The listing builds one solid part. Answer for the finished solid, in the listing's coordinates (mm). A direction names the side the tool comes from. Round coordinates to 2 decimals unless told otherwise and drop trailing zeros. Order: outer loops, then holes, each group sorted by start corner. A loop starts at its lowest first (then second) coordinate and runs counter-clockwise, first axis right, second up. Notation, with made-up numbers: (44.5, 39.5) -> (59.5, 39.5) arc R13 cw to (59.5, 62.5) -> close; hole circle Ø4 at (48.5, -6.5). An arc over 180 degrees is marked (long way). Return JSON: item names as keys, results as strings. Group by question number.
(1) Each of these flat-tipped pins is pushed along its axis until it touches: pin 1 (1.5 mm diameter, centred on x = 53.5, y = 36, fed in from +Z); pin 2 (24.5 mm diameter, centred on x = 17.5, y = 17.5, fed in from +Z); pin 3 (5 mm diameter, centred on x = 8, y = 30.5, fed in from -Z). Where does it stop, or does it pass through?
(2) Consider line 1 (X direction, y = 4, z = 15.75); line 2 (Y direction, x = 26, z = 19); line 3 (Y direction, x = 21, z = 12.25). Determine where each line is inside the solid, lowest interval first. Write a range as [from, to].
(3) Determine the mould class of faces 1 (the face through (58.55, 15, 1)), 2 (the face through (57.05, 7, 11)), 3 (the face through (-2, 30, 16)) for opening direction X: +X half, -X half, draft (parallel to the pull), parting line (faces both ways), or undercut.
(4) The part is cut by section B-B (y = 9). Determine the outline of the cut face in (x, z), plus the area to 3 significant figures.
(5) The part is cut by section D-D (y = 19.5). Determine the outline of the cut face in (x, z).
(6) The part is cut by section A-A (x = 42.5). Determine the outline of the cut face in (y, z), plus the area to 3 significant figures.
(7) Which of the six approach directions +Z, -Z, +X, -X, +Y, -Y give full straight-line access (tool end or side, diameter ignored) to faces 4 (the face through (41, 49, 16)), 5 (the face through (29, 13.5, 10)), 6 (the face through (61, 45, 16))?
(8) The part is cut by section C-C (z = 8). Count the separate pieces of the cut face and the enclosed holes in it, plus the area to 3 significant figures.
from build123d import *

# Parameters (mm, degrees)
SKETCH1_W            = 64.05
SKETCH1_H            = 52.6
BOSS_EXTRUDE1_DEPTH  = 2
SKETCH2_W            = 64.05
SKETCH2_H            = 52.6
SKETCH2_W_2          = 60.05
SKETCH2_H_2          = 48.6
BOSS_EXTRUDE2_DEPTH  = 18
SKETCH3_W            = 64.05
SKETCH3_H            = 52.6
SKETCH3_W_2          = 62.45
SKETCH3_H_2          = 51
BOSS_EXTRUDE3_DEPTH  = 2.2
SKETCH6_W            = 52.55
SKETCH6_H            = 16
CUT_EXTRUDE2_DEPTH   = 15
BOSS_EXTRUDE4_DEPTH  = 18
CUT_EXTRUDE3_DEPTH   = 3
LPATTERN1_COUNT      = 8
LPATTERN1_PITCH      = 7.6
CUT_EXTRUDE4_DEPTH   = 3
LPATTERN2_COUNT      = 5
LPATTERN2_PITCH      = 7.6
MIRROR1_COPY_1_DEPTH = 3
MIRROR1_COPY_2_DEPTH = 3
MIRROR1_COPY_3_DEPTH = 3
MIRROR1_COPY_4_DEPTH = 3
FILLET1_R            = 1
SKETCH10_W           = 52.55
SKETCH10_H           = 30
CUT_EXTRUDE5_DEPTH   = 0.2
FILLET2_R            = 2


with BuildPart() as part:
    # Sketch1 → Boss-Extrude1 (new body)
    with BuildSketch(Plane.XY):
        with Locations((29.525, 23.8)):
            Rectangle(SKETCH1_W, SKETCH1_H)
    extrude(amount=BOSS_EXTRUDE1_DEPTH)

    # Sketch2 → Boss-Extrude2 (add)
    with BuildSketch(Plane.XY.offset(2)):
        with Locations((29.525, 23.8)):
            Rectangle(SKETCH2_W, SKETCH2_H)
        with Locations((29.525, 23.8)):
            Rectangle(SKETCH2_W_2, SKETCH2_H_2, mode=Mode.SUBTRACT)
    extrude(amount=BOSS_EXTRUDE2_DEPTH)

    # Sketch3 → Boss-Extrude3 (add)
    with BuildSketch(Plane.XY.offset(20)):
        with Locations((29.525, 23.8)):
            Rectangle(SKETCH3_W, SKETCH3_H)
        with Locations((29.525, 23.8)):
            Rectangle(SKETCH3_W_2, SKETCH3_H_2, mode=Mode.SUBTRACT)
    extrude(amount=BOSS_EXTRUDE3_DEPTH)

    # Sketch6 → Cut-Extrude2 (cut)
    with BuildSketch(Plane(origin=(0, 0, 0), x_dir=(-1, 0, 0), z_dir=(0, 0, -1))):
        with Locations((-29.775, 5.5)):
            Rectangle(SKETCH6_W, SKETCH6_H)
    extrude(amount=-CUT_EXTRUDE2_DEPTH, mode=Mode.SUBTRACT)

    # Sketch7 → Boss-Extrude4 (add)
    with BuildSketch(Plane.XY.offset(2)):
        Polygon((56.05, 13.5), (56.05, -0.5), (57.05, -0.5), (57.05, 14.5), (2.5, 14.5), (2.5, -0.5), (3.5, -0.5), (3.5, 13.5), align=None)
    extrude(amount=BOSS_EXTRUDE4_DEPTH)

    # Sketch8 → Cut-Extrude3 (cut)
    with BuildSketch(Plane(origin=(0, 50.1, 0), x_dir=(1, 0, 0), z_dir=(0, 1, 0))):
        Polygon((1.5, 0), (3.5, 0), (3.3, -16), (1.7, -16), align=None)
    cut_extrude3 = extrude(amount=-CUT_EXTRUDE3_DEPTH, mode=Mode.SUBTRACT)

    # LPattern1: Cut-Extrude3 ×8
    with Locations(*[(i * LPATTERN1_PITCH, 0, 0) for i in range(1, LPATTERN1_COUNT)]):
        add(cut_extrude3, mode=Mode.SUBTRACT)

    # Sketch9 → Cut-Extrude4 (cut)
    with BuildSketch(Plane(origin=(61.55, 0, 0), x_dir=(0, 0, -1), z_dir=(1, 0, 0))):
        Polygon((0, 46.1), (0, 44.1), (-16, 44.3), (-16, 45.9), align=None)
    cut_extrude4 = extrude(amount=-CUT_EXTRUDE4_DEPTH, mode=Mode.SUBTRACT)

    # LPattern2: Cut-Extrude4 ×5
    with Locations(*[(0, -i * LPATTERN2_PITCH, 0) for i in range(1, LPATTERN2_COUNT)]):
        add(cut_extrude4, mode=Mode.SUBTRACT)

    # Mirror1: Cut-Extrude4 across plane
    add(cut_extrude4.mirror(Plane(origin=(29.525, 0, 0), x_dir=(0, 0, 1), z_dir=(1, 0, 0))), mode=Mode.SUBTRACT)

    # Mirror1 copy 1 sketch → Mirror1 copy 1 (cut)
    with BuildSketch(Plane(origin=(-2.5, -7.6, 0), x_dir=(0, 0, -1), z_dir=(-1, 0, 0))):
        Polygon((0, -46.1), (0, -44.1), (-16, -44.3), (-16, -45.9), align=None)
    extrude(amount=-MIRROR1_COPY_1_DEPTH, mode=Mode.SUBTRACT)

    # Mirror1 copy 2 sketch → Mirror1 copy 2 (cut)
    with BuildSketch(Plane(origin=(-2.5, -15.2, 0), x_dir=(0, 0, -1), z_dir=(-1, 0, 0))):
        Polygon((0, -46.1), (0, -44.1), (-16, -44.3), (-16, -45.9), align=None)
    extrude(amount=-MIRROR1_COPY_2_DEPTH, mode=Mode.SUBTRACT)

    # Mirror1 copy 3 sketch → Mirror1 copy 3 (cut)
    with BuildSketch(Plane(origin=(-2.5, -22.8, 0), x_dir=(0, 0, -1), z_dir=(-1, 0, 0))):
        Polygon((0, -46.1), (0, -44.1), (-16, -44.3), (-16, -45.9), align=None)
    extrude(amount=-MIRROR1_COPY_3_DEPTH, mode=Mode.SUBTRACT)

    # Mirror1 copy 4 sketch → Mirror1 copy 4 (cut)
    with BuildSketch(Plane(origin=(-2.5, -30.4, 0), x_dir=(0, 0, -1), z_dir=(-1, 0, 0))):
        Polygon((0, -46.1), (0, -44.1), (-16, -44.3), (-16, -45.9), align=None)
    extrude(amount=-MIRROR1_COPY_4_DEPTH, mode=Mode.SUBTRACT)

    # Fillet1
    fillet1_edges = [part.edges().sort_by_distance(p)[0] for p in [
        (56.05, 13.5, 10),
        (3.5, 13.5, 10),
        (3.5, -2.5, 7.5),
        (56.05, -2.5, 7.5),
        (-2.5, 50.1, 11.1),
        (61.55, 50.1, 11.1),
        (61.55, -2.5, 11.1),
        (-2.5, -2.5, 11.1),
    ]]
    fillet(fillet1_edges, radius=FILLET1_R)

    # Sketch10 → Cut-Extrude5 (cut)
    with BuildSketch(Plane(origin=(0, 0, 0), x_dir=(-1, 0, 0), z_dir=(0, 0, -1))):
        with Locations((-29.775, 30.5)):
            Rectangle(SKETCH10_W, SKETCH10_H)
    extrude(amount=-CUT_EXTRUDE5_DEPTH, mode=Mode.SUBTRACT)

    # Fillet2
    fillet2_edges = [part.edges().sort_by_distance(p)[0] for p in [
        (3.5, 45.5, 0.1),
        (3.5, 15.5, 0.1),
        (56.05, 15.5, 0.1),
        (56.05, 45.5, 0.1),
    ]]
    fillet(fillet2_edges, radius=FILLET2_R)


solid = part.part
Answer below:
{
 "1": {"pin 1": "stops at z = 2", "pin 2": "stops at z = 20", "pin 3": "stops at z = 0.2"},
 "2": {"line 1": "x = [-2.5, -0.5], [2.5, 3.5], [56.05, 57.05], [59.55, 61.55]", "line 2": "y = [-2.5, -0.5], [13.5, 14.5], [48.1, 50.1]", "line 3": "y = [13.5, 14.5], [48.1, 50.1]"},
 "3": {"face 1": "+X half", "face 2": "undercut", "face 3": "draft"},
 "4": {"outline": "(-2.5, 0) -> (3.5, 0) -> (3.5, 20) -> (2.5, 20) -> (2.5, 2) -> (-0.5, 2) -> (-0.5, 20) -> (-1.7, 20) -> (-1.7, 22.2) -> (-2.5, 22.2) -> close; (56.05, 0) -> (61.55, 0) -> (61.55, 22.2) -> (60.75, 22.2) -> (60.75, 20) -> (59.55, 20) -> (59.55, 2) -> (57.05, 2) -> (57.05, 20) -> (56.05, 20) -> close", "area": "135 mm²"},
 "5": {"outline": "(-2.5, 0) -> (3.5, 0) -> (3.5, 0.2) -> (56.05, 0.2) -> (56.05, 0) -> (61.55, 0) -> (61.55, 22.2) -> (60.75, 22.2) -> (60.75, 20) -> (59.55, 20) -> (59.55, 2) -> (-0.5, 2) -> (-0.5, 20) -> (-1.7, 20) -> (-1.7, 22.2) -> (-2.5, 22.2) -> close"},
 "6": {"outline": "(-2.5, 15) -> (-0.5, 15) -> (-0.5, 20) -> (-1.7, 20) -> (-1.7, 22.2) -> (-2.5, 22.2) -> close; (13.5, 0) -> (15.5, 0) -> (15.5, 0.2) -> (45.5, 0.2) -> (45.5, 0) -> (50.1, 0) -> (50.1, 22.2) -> (49.3, 22.2) -> (49.3, 20) -> (48.1, 20) -> (48.1, 2) -> (14.5, 2) -> (14.5, 20) -> (13.5, 20) -> close", "area": "135 mm²"},
 "7": {"face 4": "-Z, +Y", "face 5": "+Z, -Z", "face 6": "-Z, +X, -X"},
 "8": {"separate pieces": "18", "enclosed holes": "0", "area": "362 mm²"}
}
